from build123d import *
from build123d.topology import SkipClean

# Parameters (mm, degrees)
SKETCH1_R      = 0.75
SKETCH1_R_2    = 1.5
EXTRUDE1_DEPTH = 1.5
SKETCH2_R      = 0.75
SKETCH2_R_2    = 1.5
EXTRUDE2_DEPTH = 2
SKETCH3_R      = 5
SKETCH3_R_2    = 1.5
EXTRUDE3_DEPTH = 3


with BuildPart() as part:
    # Sketch1 → Extrude1 (new body, symmetric)
    with BuildSketch(Plane(origin=(0, 0, 0), x_dir=(1, 0, 0), z_dir=(0, 1, 0))):
        with BuildLine():
            Line((-30, 2.5), (30, 2.5))
            ThreePointArc((30, 2.5), (32.440660221, 0.541458851), (31.057213663, -2.26545785))
            Line((31.057213663, -2.26545785), (1.057213663, -16.26545785))
            ThreePointArc((1.057213663, -16.26545785), (0, -16.5), (-1.057213663, -16.26545785))
            Line((-1.057213663, -16.26545785), (-31.057213663, -2.26545785))
            ThreePointArc((-31.057213663, -2.26545785), (-32.440660221, 0.541458851), (-30, 2.5))
        make_face()
        with Locations(Location((30, 0, 0), (0, 0, 270))):  # turned: the seam where the file's is
            Circle(SKETCH1_R, mode=Mode.SUBTRACT)
        with Locations(Location((-30, 0, 0), (0, 0, 270))):  # turned: the seam where the file's is
            Circle(SKETCH1_R, mode=Mode.SUBTRACT)
        with Locations(Location((0, -14, 0), (0, 0, 270))):  # turned: the seam where the file's is
            Circle(SKETCH1_R_2, mode=Mode.SUBTRACT)
        with Locations(Location((0, 0, 0), (0, 0, 270))):  # turned: the seam where the file's is
            Circle(SKETCH1_R_2, mode=Mode.SUBTRACT)
    extrude(amount=EXTRUDE1_DEPTH, both=True)

    # Sketch2 → Extrude2 (add, symmetric)
    with SkipClean():  # keep this step's faces unmerged: merging them makes the solid invalid here
        with BuildSketch(Plane(origin=(0, 0, 0), x_dir=(1, 0, 0), z_dir=(0, 1, 0))):
            with BuildLine():
                Line((-27.272821971, 1.25), (-0.829156198, 1.25))
                ThreePointArc((-0.829156198, 1.25), (0, -1.5), (0.829156198, 1.25))
                Line((0.829156198, 1.25), (27.272821971, 1.25))
                ThreePointArc((27.272821971, 1.25), (33, 0), (27.272821971, -1.25))
                Line((27.272821971, -1.25), (3, -1.25))
                Line((3, -1.25), (3, -14))
                ThreePointArc((3, -14), (0, -17), (-3, -14))
                Line((-3, -14), (-3, -1.25))
                Line((-3, -1.25), (-27.272821971, -1.25))
                ThreePointArc((-27.272821971, -1.25), (-33, 0), (-27.272821971, 1.25))
            make_face()
            with Locations(Location((30, 0, 0), (0, 0, 270))):  # turned: the seam where the file's is
                Circle(SKETCH2_R, mode=Mode.SUBTRACT)
            with Locations(Location((0, -14, 0), (0, 0, 270))):  # turned: the seam where the file's is
                Circle(SKETCH2_R_2, mode=Mode.SUBTRACT)
            with Locations(Location((-30, 0, 0), (0, 0, 270))):  # turned: the seam where the file's is
                Circle(SKETCH2_R, mode=Mode.SUBTRACT)
        extrude(amount=EXTRUDE2_DEPTH, both=True)

    # Sketch3 → Extrude3 (add, symmetric)
    with SkipClean():  # keep this step's faces unmerged: merging them makes the solid invalid here
        with BuildSketch(Plane(origin=(0, 0, 0), x_dir=(1, 0, 0), z_dir=(0, 1, 0))):
            with Locations(Location((0, 0, 0), (0, 0, 270))):  # turned: the seam where the file's is
                Circle(SKETCH3_R)
            with Locations(Location((0, 0, 0), (0, 0, 270))):  # turned: the seam where the file's is
                Circle(SKETCH3_R_2, mode=Mode.SUBTRACT)
        extrude(amount=EXTRUDE3_DEPTH, both=True)


solid = part.part
CAD build for the part. Positions are in the model's coordinates, mm. A direction names the side the tool comes from. Round coordinates to 2 decimals unless told otherwise and drop trailing zeros. Write each loop counter-clockwise with the first axis right and the second up, starting at its lowest first coordinate (ties: lowest second). Pieces come first, ordered by that corner, then holes. Notation, with made-up numbers: M 75,80.5 L 105,80.5 A20 cw 105,97.5 Z; hole C 22.5,86.5 d10. An arc over 180 degrees is marked long. Put each result on its own line as item: value. Start each with the question number.
1) Saw through at D-D, the plane z = 7.5. Write the cut outline in (x, y), and give its area (3 significant figures).
2) Saw through at A-A, the plane z = 0. Write the cut outline in (x, y), and give its area (3 significant figures).
3) Pin check, flat tips, straight feed: pin 1 Ø1 at (x, z) = (-11, -1.5) entering from -Y; pin 2 Ø8 at (x, z) = (19, 7.5) entering from -Y; pin 3 Ø0.6 at (x, z) = (-17.5, -2) entering from +Y; pin 4 Ø3 at (y, z) = (-1, -0.5) entering from -X. Stop position of each tip, or through.
4) Saw through at C-C, the plane x = 10. Write the cut outline in (y, z).
5) 3-axis set-ups, long thin cutter, end or side, ignore diameter. For faces 1 (the flat face through (16, 0, -2.5)), 2 (the flat face through (17, 1.5, -2)), 3 (the flat face through (-13, 1.5, 7)), 4 (the flat face through (17, -1.5, -2)): which of +Z, -Z, +X, -X, +Y, -Y reach the whole face in a straight line?
6) Pull direction X, two halves, no side cores. Call faces 5 (the flat face through (13, -1.5, 7)), 6 (the flat face through (0, -2, 10)), 7 (the flat face through (-13, -1.5, 7)), 8 (the cylindrical face through (0, 0, 17)): pulls with the +X half, pulls with the -X half, needs draft (parallel to the pull), parting line crosses it, or undercut.
7) Saw through at B-B, the plane y = -0.9. Write the cut outline in (x, z).
8) Drill centre lines: probe 1 along X at (y, z) = (-1.7, 0); probe 2 along X at (y, z) = (-0.6, 14); probe 3 along Z at (x, y) = (-0.5, -1.8). Where is each one in solid material? Low to high. Write a range as [from, to].
Resolved:
1. outline: M -19.84,-1.5 L -3,-1.5 L -3,-2 L 3,-2 L 3,-1.5 L 19.84,-1.5 L 19.84,1.5 L 3,1.5 L 3,2 L -3,2 L -3,1.5 L -19.84,1.5 Z
1. area: 125 mm²
2. outline: M -33,-2 L -30.75,-2 L -30.75,2 L -33,2 Z; M -29.25,-2 L -5,-2 L -5,-3 L -1.5,-3 L -1.5,3 L -5,3 L -5,2 L -29.25,2 Z; M 1.5,-3 L 5,-3 L 5,-2 L 29.25,-2 L 29.25,2 L 5,2 L 5,3 L 1.5,3 Z; M 30.75,-2 L 33,-2 L 33,2 L 30.75,2 Z
2. area: 254 mm²
3. pin 1: y = -2
3. pin 2: y = -1.5
3. pin 3: y = 1.5
3. pin 4: x = -33
4. outline: M -2,-1.25 L -1.5,-1.25 L -1.5,-2.5 L 1.5,-2.5 L 1.5,-1.25 L 2,-1.25 L 2,1.25 L 1.5,1.25 L 1.5,12.09 L -1.5,12.09 L -1.5,1.25 L -2,1.25 Z
5. face 1: -Z, +Y, -Y
5. face 2: -Z, +Y
5. face 3: +Z, +Y
5. face 4: -Z, -Y
6. face 5: undercut
6. face 6: needs draft
6. face 7: undercut
6. face 8: parting line crosses it
7. outline: M -29.55,2.97 A3 ccw long -28.34,-2.5 L -4.33,-2.5 A5 ccw 4.33,-2.5 L 28.34,-2.5 A3 ccw long 29.55,2.97 L 2.56,15.56 A3 ccw -2.56,15.56 Z; hole C -30,0 d1.5; hole C 0,0 d3; hole C 0,14 d3; hole C 30,0 d1.5
8. probe 1: [-33, -30.75], [-29.25, -1.5], [1.5, 29.25], [30.75, 33]
8. probe 2: [-5.91, -1.5], [1.5, 5.91]
8. probe 3: [-4.97, -1.41], [1.41, 12.59], [15.41, 16.96]
